```python
from build123d import *

# Parameters (mm, degrees)
BOSS_EXTRUDE1_DEPTH = 0.840608912
SKETCH2_R           = 11.136118556
BOSS_EXTRUDE2_DEPTH = 50.8
SKETCH3_W           = 86.137031446
SKETCH3_H           = 59.748072355
BOSS_EXTRUDE3_DEPTH = 50.8
CUT_EXTRUDE1_DEPTH  = 109.100560925


with BuildPart() as part:
    # Sketch1 → Boss-Extrude1 (new body)
    with BuildSketch(Plane.XY):
        with BuildLine():
            Line((-11.136118556, 0), (-11.136118556, 25.4))
            Line((-11.136118556, 25.4), (11.136118556, 25.4))
            Line((11.136118556, 25.4), (11.136118556, 0))
            ThreePointArc((11.136118556, 0), (0, 11.136118556), (-11.136118556, 0))
        make_face()
    extrude(amount=BOSS_EXTRUDE1_DEPTH)

    # Sketch2 → Boss-Extrude2 (add)
    with BuildSketch(Plane.XY):
        Circle(SKETCH2_R)
    extrude(amount=BOSS_EXTRUDE2_DEPTH)

    # Sketch3 → Boss-Extrude3 (add)
    with BuildSketch(Plane.XY):
        with Locations((0, 55.274036178)):
            Rectangle(SKETCH3_W, SKETCH3_H)
    extrude(amount=BOSS_EXTRUDE3_DEPTH)

    # Sketch4 → Cut-Extrude1 (cut, through all)
    with BuildSketch(Plane.XY.offset(50.8)):
        Polygon((20.431484277, 85.148072355), (20.431484277, 59.748072355), (31.75, 59.748072355), (31.75, 34.29), (-31.75, 34.29), (-31.75, 59.748072355), (-20.431484277, 59.748072355), (-20.431484277, 85.148072355), align=None)
    extrude(amount=-CUT_EXTRUDE1_DEPTH, mode=Mode.SUBTRACT)


solid = part.part
```
The model under review builds one solid part; all positions refer to its coordinate system, in mm. A direction names the side the tool comes from. Round coordinates to 2 decimals unless told otherwise and drop trailing zeros. Order: outer loops, then holes, each group sorted by start corner. A loop starts at its lowest first (then second) coordinate and runs counter-clockwise, first axis right, second up. Notation, with made-up numbers: (26, 63) -> (48, 63) arc R17 cw to (48, 81) -> close; hole circle Ø3 at (59, -25). An arc over 180 degrees is marked (long way). One line per item, written item: value. Start each with the question number.
Q1. Take a section at C-C (x = -30.5). Write out the cut boundary in (y, z).
Q2. Mouldability with a two-part tool opening along X and no side actions: class faces 1 (the face through (0, 0, 50.8)), 2 (the face through (0, 34.29, 26)), 3 (the face through (-8.837, -6.776, 25.044)), 4 (the face through (26, 59.748, 26)) as released by +X, released by -X, zero draft, split by the parting line, or undercut.
Q3. Take a section at A-A (z = 6). Write out the cut boundary in (x, y).
Q4. Clearance check with flat-ended pins moving along their axes: pin 1 Ø10 at (x, y) = (4.5, 6) entering from -Z; pin 2 Ø15 at (x, z) = (-3, 17) entering from +Y; pin 3 Ø2 at (x, z) = (24.5, 28.5) entering from -Y; pin 4 Ø1.5 at (y, z) = (0.5, 43.5) entering from -X. State where each tip first meets the part, or that it passes through.
Q5. Wall thickness on line 1 (X direction, y = 80, z = 33); line 2 (Y direction, x = 20.5, z = 21.5); line 3 (X direction, y = 44.5, z = 17): over which ranges is each line inside the solid? List them lowest first.
Q6. Take a section at B-B (y = 64.5). Write out the cut boundary in (x, z), and give its area (3 significant figures).
Q7. Take a section at D-D (x = 0). Write out the cut boundary in (y, z).
Q8. Machinability: for faces 5 (the face through (-32, 85.148, 25)), 6 (the face through (-31.75, 47, 26)), 7 (the face through (-20.431, 72, 26)), which of the approach directions +Z, -Z, +X, -X, +Y, -Y give a long, thin tool a straight path to every point of the face, cutting with its end or side? Answer none if there is none.
Reported:
1. outline: (25.4, 0) -> (34.29, 0) -> (34.29, 50.8) -> (25.4, 50.8) -> close; (59.75, 0) -> (85.15, 0) -> (85.15, 50.8) -> (59.75, 50.8) -> close
2. face 1: zero draft
2. face 2: undercut
2. face 3: split by the parting line
2. face 4: undercut
3. outline: (-43.07, 25.4) -> (43.07, 25.4) -> (43.07, 85.15) -> (20.43, 85.15) -> (20.43, 59.75) -> (31.75, 59.75) -> (31.75, 34.29) -> (-31.75, 34.29) -> (-31.75, 59.75) -> (-20.43, 59.75) -> (-20.43, 85.15) -> (-43.07, 85.15) -> close; circle Ø22.27 at (0, 0)
4. pin 1: stops at z = 0
4. pin 2: stops at y = 34.29
4. pin 3: stops at y = 25.4
4. pin 4: stops at x = -11.14
5. line 1: x = -43.07 to -20.43, 20.43 to 43.07
5. line 2: y = 25.4 to 34.29, 59.75 to 85.15
5. line 3: x = -43.07 to -31.75, 31.75 to 43.07
6. outline: (-43.07, 0) -> (-20.43, 0) -> (-20.43, 50.8) -> (-43.07, 50.8) -> close; (20.43, 0) -> (43.07, 0) -> (43.07, 50.8) -> (20.43, 50.8) -> close
6. area: 2,300 mm2
7. outline: (-11.14, 0) -> (34.29, 0) -> (34.29, 50.8) -> (25.4, 50.8) -> (25.4, 0.84) -> (11.14, 0.84) -> (11.14, 50.8) -> (-11.14, 50.8) -> close
8. face 5: +Z, -Z, +X, -X, +Y
8. face 6: +Z, -Z
8. face 7: +Z, -Z, +Y
